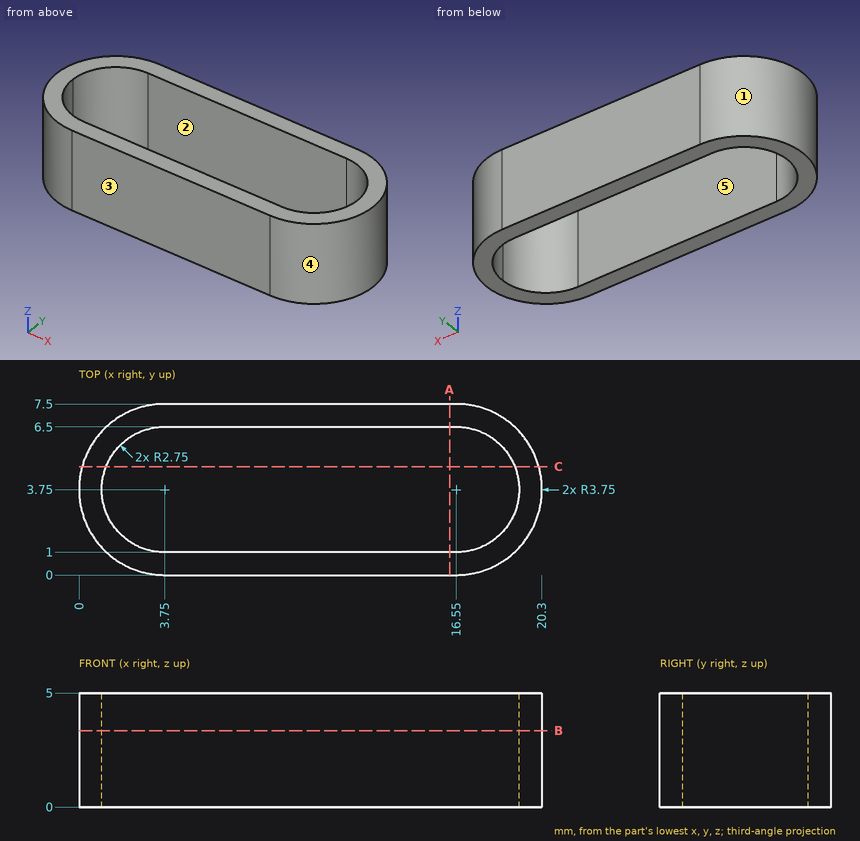
Input: dimensioned drawing with shaded views. Units: mm. Origin: part minimum x, y, z. A direction names the side the tool comes from. Round coordinates to 2 decimals unless told otherwise and drop trailing zeros. Loops run counter-clockwise (first coordinate to the right, second up) from the corner with the lowest first, then second, coordinate; pieces in that order, holes last. Notation, with made-up numbers: (60.5, -34) -> (70.5, -34) arc R21 cw to (70.5, -21) -> close; hole circle Ø10 at (-13, -38.5). An arc over 180 degrees is marked (long way). Use one line per item in the form item = value. Start each with the question number.
1) First-contact query: P1, Ø2, axis at x = 17.5, z = 0.5, coming from the -Y side; P2, Ø1, axis at y = 2.5, z = 3, coming from the +X side; P3, Ø3, axis at x = 9.5, y = 3.5, coming from the -Z side. Flat tips, straight axial feed; report the tip coordinate or a pass-through.
2) Section C-C on y = 4.75. Output: boundary loops of the cut face in (x, z).
3) Access query for the marked faces 1 and 2. Directions: +Z, -Z, +X, -X, +Y, -Y. A direction counts if a zero-diameter tool reaches every point of the face in a straight line with its end or side. Return the directions, or none.
4) Section B-B on z = 3.35. Output: boundary loops of the cut face in (x, y).
5) Draft query along X for the marked faces 3, 4 and 5. Return one class per face: released by +X, released by -X, zero draft, split by the parting line, or undercut.
6) Line query: L1, parallel to Y at x = 11.75, z = 1; L2, parallel to X at y = 2, z = 3; L3, parallel to X at y = 4.75, z = 2.55. Output: solid intervals per line, ascending.
7) Section A-A on x = 16.25. Output: boundary loops of the cut face in (y, z).
Response:
q1.P1 = 0
q1.P2 = 20.22
q1.P3 = through
q2.outline = (0.14, 0) -> (1.19, 0) -> (1.19, 5) -> (0.14, 5) -> close; (19.11, 0) -> (20.16, 0) -> (20.16, 5) -> (19.11, 5) -> close
q3.face_1 = +Z, -Z, -X
q3.face_2 = +Z, -Z
q4.outline = (3.75, 0) -> (16.55, 0) arc R3.75 ccw to (16.55, 7.5) -> (3.75, 7.5) arc R3.75 ccw to start; hole (3.75, 1) -> (16.55, 1) arc R2.75 ccw to (16.55, 6.5) -> (3.75, 6.5) arc R2.75 ccw to start
q5.face_3 = zero draft
q5.face_4 = released by +X
q5.face_5 = undercut
q6.L1 = 0 to 1, 6.5 to 7.5
q6.L2 = 0.43 to 1.63, 18.67 to 19.87
q6.L3 = 0.14 to 1.19, 19.11 to 20.16
q7.outline = (0, 0) -> (1, 0) -> (1, 5) -> (0, 5) -> close; (6.5, 0) -> (7.5, 0) -> (7.5, 5) -> (6.5, 5) -> close
